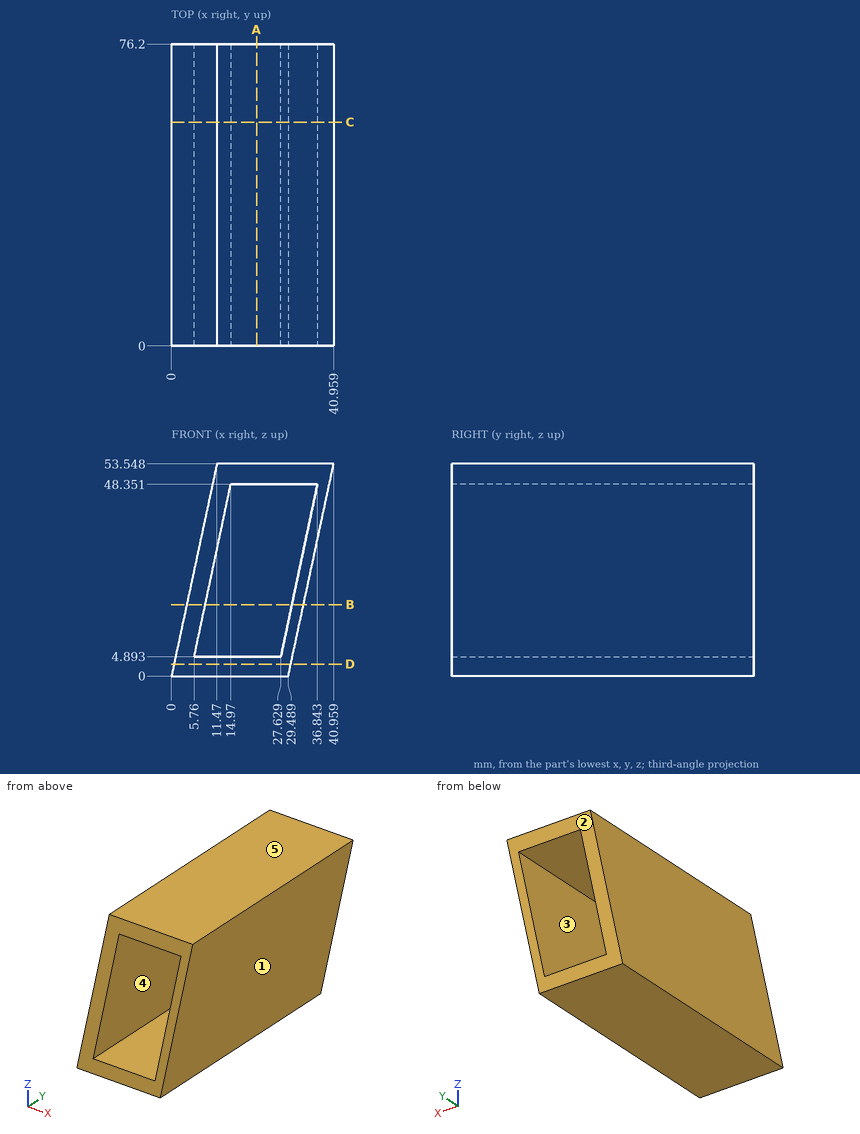
Geometry check sheet. Reference: drawing and pictorial views, mm from the part's lowest x, y, z. A direction names the side the tool comes from. Coordinates: 2 decimals unless noted, no trailing zeros. Write each loop counter-clockwise with the first axis right and the second up, starting at its lowest first coordinate (ties: lowest second). Pieces come first, ordered by that corner, then holes. Notation, with made-up numbers: (88.5, 56.25) - (133.5, 56.25) arc R32 ccw to (133.5, 89.25) - close; hole circle Ø7 at (18, -32.5). An arc over 180 degrees is marked (long way). One line per question, with ' | ' between items. Start each with the question number.
1. Access from +Z, -Z, +X, -X, +Y, -Y to the whole of each face (thin tool, end or side, straight path). Record for the marked faces 4 and 5.
2. Section check D-D (z = 3). Enter the section's corners in (x, y), plus the area to 3 significant figures.
3. Material ranges on line 1 along Z through (x, y) = (19, 14.5); line 2 along X through (y, z) = (10, 9); line 3 along X through (y, z) = (49, 47), recorded low to high.
4. Section check B-B (z = 18). Enter the section's corners in (x, y) (1 decimal).
5. Gauge pin test, flat ends, axial feed: P1, Ø2, axis at y = 18.5, z = 31.5, coming from the +X side; P2, Ø8, axis at y = 25, z = 23.5, coming from the -X side; P3, Ø8, axis at y = 22.5, z = 6, coming from the -X side. Record the tip position at first contact, or that the pin passes through.
6. Section check C-C (y = 56.5). Enter the section's corners in (x, z).
7. Section check A-A (x = 21.5). Enter the section's corners in (y, z).
8. Draft check along X on the marked faces 1, 2 and 3. Enter one of: released by +X, released by -X, zero draft, split by the parting line, or undercut.
Computed values:
1) face 4: +Y, -Y | face 5: +Z, +X, -X, +Y, -Y
2) outline: (0.64, 0) - (30.13, 0) - (30.13, 76.2) - (0.64, 76.2) - close | area: 2,250 mm²
3) line 1: 0 to 4.89, 48.35 to 53.55 | line 2: 1.93 to 6.63, 28.5 to 31.42 | line 3: 10.07 to 14.68, 36.56 to 39.56
4) outline: (3.9, 0) - (8.5, 0) - (8.5, 76.2) - (3.9, 76.2) - close; (30.4, 0) - (33.3, 0) - (33.3, 76.2) - (30.4, 76.2) - close
5) P1: x = 36.45 | P2: x = 4.18 | P3: x = 0.43
6) outline: (0, 0) - (29.49, 0) - (40.96, 53.55) - (11.47, 53.55) - close; hole (5.76, 4.89) - (27.63, 4.89) - (36.84, 48.35) - (14.97, 48.35) - close
7) outline: (0, 0) - (76.2, 0) - (76.2, 4.89) - (0, 4.89) - close; (0, 48.35) - (76.2, 48.35) - (76.2, 53.55) - (0, 53.55) - close
8) face 1: released by +X | face 2: zero draft | face 3: undercut
